Study the drawing (mm; zero at the part's minimum x, y, z) and answer. A direction names the side the tool comes from. Coordinates: 2 decimals unless noted, no trailing zeros. Order: outer loops, then holes, each group sorted by start corner. A loop starts at its lowest first (then second) coordinate and runs counter-clockwise, first axis right, second up.
1. Flat-ended cylindrical pins translate along their axes: pin 1 Ø0.8 at (y, z) = (3.5, 2.5) entering from +X; pin 2 Ø1.8 at (x, y) = (4.5, 3) entering from -Z; pin 3 Ø1.3 at (y, z) = (2, 5) entering from +X. Find the tip coordinate at first contact, or state that the pin passes through.
2. Find the intervals of material crossed by probe 1 along X at (y, z) = (3.2, 2); probe 2 along X at (y, z) = (4, 3.75); probe 3 along Z at (x, y) = (6, 1.35), in increasing order.
3. A tool of negligible diameter and unlimited length cuts with its end or side. For the marked faces 1, 2, 3 and 4, from which of +Z, -Z, +X, -X, +Y, -Y can it reach the whole face along a straight path? Write none if from no direction.
4. The part is cut by section C-C, the plane x = 3.75. Give the vertices of the cut face in (y, z), then the cut area to 3 significant figures.
5. Determine the mould class of the marked faces 5, 6 and 7 for opening direction Y: +Y half, -Y half, draft (parallel to the pull), parting line (faces both ways), or undercut.
6. The part is cut by section D-D, the plane x = 7.25. Give the vertices of the cut face in (y, z).
7. The part is cut by section B-B, the plane z = 4. Give the vertices of the cut face in (x, y), then the cut area to 3 significant figures.
8. The part is cut by section A-A, the plane x = 1.1. Give the vertices of the cut face in (y, z), then the cut area to 3 significant figures.
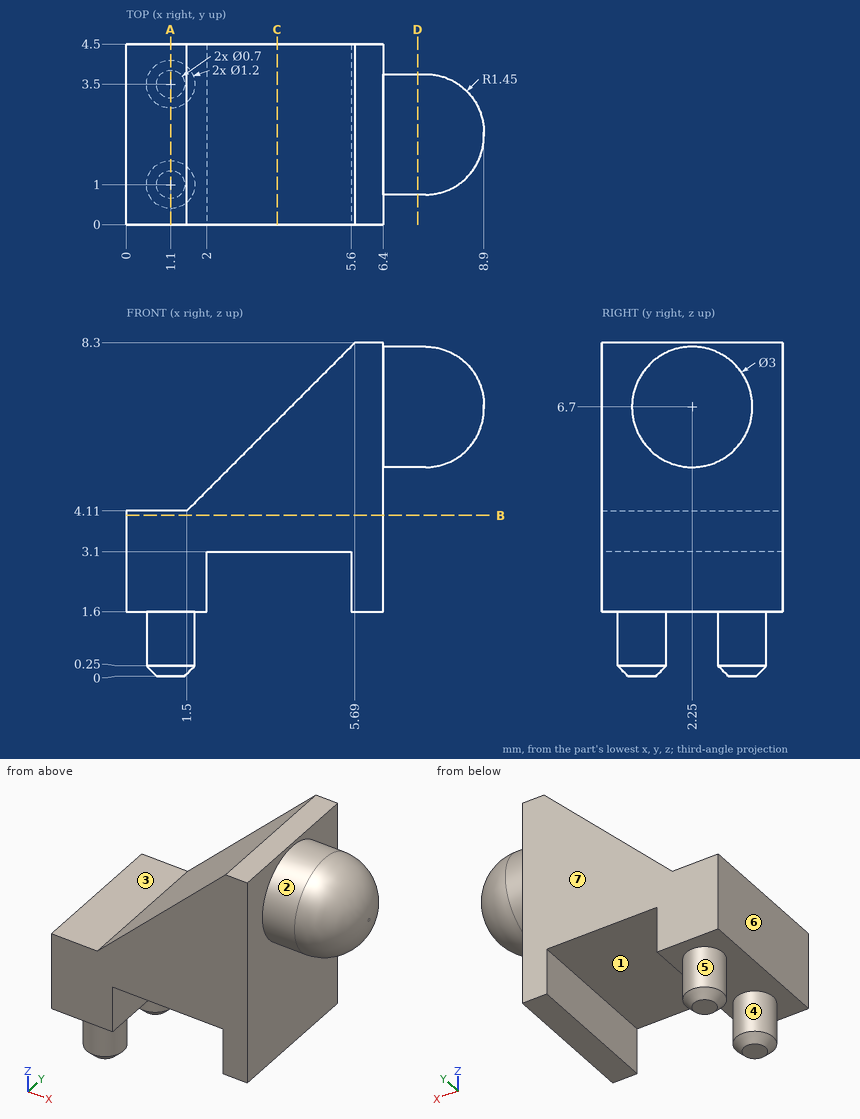
Geometry says:
1. pin 1: stops at x = 6.4
1. pin 2: stops at z = 3.1
1. pin 3: stops at x = 8.48
2. probe 1: x = 0 to 2, 5.6 to 6.4
2. probe 2: x = 0 to 6.4
2. probe 3: z = 1.6 to 8.3
3. face 1: -Z, +Y, -Y
3. face 2: +X
3. face 3: +Z, -X, +Y, -Y
3. face 4: -Z
4. outline: (0, 3.1) - (4.5, 3.1) - (4.5, 6.36) - (0, 6.36) - close
4. area: 14.7 mm2
5. face 5: undercut
5. face 6: draft
5. face 7: +Y half
6. outline: circle Ø3 at (2.25, 6.7)
7. outline: (0, 0) - (6.4, 0) - (6.4, 4.5) - (0, 4.5) - close
7. area: 28.8 mm2
8. outline: (0, 1.6) - (0.4, 1.6) - (0.4, 0.25) - (0.65, 0) - (1.35, 0) - (1.6, 0.25) - (1.6, 1.6) - (2.9, 1.6) - (2.9, 0.25) - (3.15, 0) - (3.85, 0) - (4.1, 0.25) - (4.1, 1.6) - (4.5, 1.6) - (4.5, 4.11) - (0, 4.11) - close
8. area: 15.0 mm2
